Here's how the part is built. I have some questions about the finished solid (model axes, mm). A direction names the side the tool comes from. Round coordinates to 2 decimals unless told otherwise and drop trailing zeros. Answer in a Markdown table with one row per item. Add a question column.
from build123d import *

# Parameters (mm, degrees)
F_1_4_CLEARANCE_HOLE1_D = 6.35


with BuildPart() as part:
    # Sketch1 → Revolve1 (revolve)
    with BuildSketch(Plane(origin=(0, 0, 0), x_dir=(0, 0, -1), z_dir=(1, 0, 0))):
        with BuildLine():
            Line((23.142718313, -40.383438187), (26.454877971, -39.495947681))
            Line((26.454877971, -39.495947681), (28.75042701, -36.777175972))
            Line((28.75042701, -36.777175972), (28.719920063, -36.663322494))
            ThreePointArc((28.719920063, -36.663322494), (33.876569057, -37.507311548), (37.920363558, -34.198071089))
            Line((37.920363558, -34.198071089), (37.950870506, -34.311924567))
            Line((37.950870506, -34.311924567), (41.298260144, -35.518675415))
            Line((41.298260144, -35.518675415), (44.610419802, -34.63118491))
            Line((44.610419802, -34.63118491), (42.966918866, -28.497555913))
            Line((42.966918866, -28.497555913), (36.833289869, -30.141056849))
            Line((36.833289869, -30.141056849), (37.655040337, -33.207871348))
            Line((37.655040337, -33.207871348), (28.454596842, -35.673122752))
            Line((28.454596842, -35.673122752), (27.632846373, -32.606308254))
            Line((27.632846373, -32.606308254), (21.499217376, -34.24980919))
            Line((21.499217376, -34.24980919), (23.142718313, -40.383438187))
        make_face()
    revolve(axis=Axis((0, -34.24980919, -21.499217376), (0, 0.258819045102523, -0.9659258262890678)))

    # 1/4 Clearance Hole1 (through all)
    with Locations(Plane(origin=(0, 3.080502166, -11.496590595), x_dir=(1, 0, 0), z_dir=(0, -0.25881904510252046, 0.9659258262890684))):
        with Locations((0, -38.647182154)):
            Hole(F_1_4_CLEARANCE_HOLE1_D / 2)


solid = part.part
Item 1: If we mould it in two halves opening along Z, with no side actions, what happens to faces 1 (the conical face through (1.7, -34.06, -38.07)), 2 (the flat face through (2.733, -31.138, -43.674)), 3 (the cylindrical face through (-1.91, -39.65, -24.75))? For each: pulls with the +Z half, pulls with the -Z half, needs draft (parallel to the pull), parting line crosses it, or undercut.
Item 2: I need wall thicknesses on line 1 along X through (y, z) = (-32.25, -24); line 2 along Y through (x, z) = (-2.75, -23.75); line 3 along Y through (x, z) = (-2.5, -35.5). Which ranges of each line are inside material? Lowest first, please. Write a range as from..to.
Item 3: If we section it at A-A on x = 4.75: Give the number of separate pieces and of enclosed holes in the cut face, then the cut area to 3 significant figures.
Item 4: For P1, Ø2, axis at x = -4.5, z = -38.5, coming from the +Y side; P2, Ø1, axis at y = -34, z = -33, coming from the +X side; P3, Ø1, axis at x = 0, z = -28.5, coming from the +Y side, each with a flat end and sliding along its axis, tell me the tip position at first contact or that it passes through.
Item 5: On a 3-axis mill with a long thin cutter (end or side, diameter ignored), from which of +Z, -Z, +X, -X, +Y, -Y can I reach the whole of each face in a straight line? I mean faces 4 (the flat face through (2.73, -31.61, -20.79)), 5 (the conical face through (-1.327, -36.712, -28.586)). Say none if no direction works.
Results list:
| question | item | result |
|---|---|---|
| 1 | face 1 | undercut |
| 1 | face 2 | pulls with the -Z half |
| 1 | face 3 | parting line crosses it |
| 2 | line 1 | -6.22..-2.9, 2.9..6.22 |
| 2 | line 2 | -39.57..-35.29, -32..-28.01 |
| 2 | line 3 | -36.21..-32.52, -28.47..-26.54 |
| 3 | separate pieces | 3 |
| 3 | enclosed holes | 0 |
| 3 | area | 139 mm² |
| 4 | P1 | y = -24.16 |
| 4 | P2 | x = 5.94 |
| 4 | P3 | y = -25.91 |
| 5 | face 4 | +Z, +X, -X, -Y |
| 5 | face 5 | none |
